Check sheet for the modelled part. Datum: model origin and axes. Units: mm. A direction names the side the tool comes from. Round coordinates to 2 decimals unless told otherwise and drop trailing zeros. Order: outer loops, then holes, each group sorted by start corner. A loop starts at its lowest first (then second) coordinate and runs counter-clockwise, first axis right, second up. Notation, with made-up numbers: (32.25, -36.5) -> (64.25, -36.5) arc R24 ccw to (64.25, -7.5) -> close; hole circle Ø5 at (60.25, -34). An arc over 180 degrees is marked (long way). Answer as CSV lines item,"result". Start each with the question number.
from build123d import *

# Parameters (mm, degrees)
SKICA1_W                 = 120
SKICA1_H                 = 75
P_IDAT_VYSUNUT_M9_DEPTH  = 7
SKICA9_W                 = 60
SKICA9_H                 = 75
P_IDAT_VYSUNUT_M10_DEPTH = 7
SKICA10_W                = 60
SKICA10_H                = 75
P_IDAT_VYSUNUT_M11_DEPTH = 7
SKICA11_W                = 120
SKICA11_H                = 60
P_IDAT_VYSUNUT_M12_DEPTH = 7
SKICA12_W                = 120
SKICA12_H                = 60
P_IDAT_VYSUNUT_M13_DEPTH = 7
SKICA13_R                = 1.75
SKICA13_W                = 7.3
SKICA13_H                = 8.5
ODEBRAT_VYSUNUT_M1_DEPTH = 7


with BuildPart() as part:
    # Skica1 → Přidat vysunutím9 (new body)
    with BuildSketch(Plane.XY):
        Rectangle(SKICA1_W, SKICA1_H)
    extrude(amount=P_IDAT_VYSUNUT_M9_DEPTH)

    # Skica9 → Přidat vysunutím10 (add)
    with BuildSketch(Plane.ZY.offset(60)):
        with Locations((30, 0)):
            Rectangle(SKICA9_W, SKICA9_H)
    extrude(amount=-P_IDAT_VYSUNUT_M10_DEPTH)

    # Skica10 → Přidat vysunutím11 (add)
    with BuildSketch(Plane(origin=(60, 0, 0), x_dir=(0, 0, -1), z_dir=(1, 0, 0))):
        with Locations((-30, 0)):
            Rectangle(SKICA10_W, SKICA10_H)
    extrude(amount=-P_IDAT_VYSUNUT_M11_DEPTH)

    # Skica11 → Přidat vysunutím12 (add)
    with BuildSketch(Plane(origin=(0, -37.5, 0), x_dir=(-1, 0, 0), z_dir=(0, -1, 0))):
        with Locations((0, -30)):
            Rectangle(SKICA11_W, SKICA11_H)
    extrude(amount=-P_IDAT_VYSUNUT_M12_DEPTH)

    # Skica12 → Přidat vysunutím13 (add)
    with BuildSketch(Plane(origin=(0, 37.5, 0), x_dir=(1, 0, 0), z_dir=(0, 1, 0))):
        with Locations((0, -30)):
            Rectangle(SKICA12_W, SKICA12_H)
    extrude(amount=-P_IDAT_VYSUNUT_M13_DEPTH)

    # Skica13 → Odebrat vysunutím1 (cut)
    with BuildSketch(Plane.ZY.offset(60)):
        with Locations(Location((41.3, 13.25, 0), (0, 0, 270))):
            Circle(SKICA13_R)
        with Locations((12.65, 13.25)):
            Rectangle(SKICA13_W, SKICA13_H)
    extrude(amount=-ODEBRAT_VYSUNUT_M1_DEPTH, mode=Mode.SUBTRACT)


solid = part.part
1) Depth check by flat-ended pin: pin 1 Ø18.5 at (x, y) = (-18.5, -3.5) entering from +Z. Enter the tip coordinate at first touch or a pass-through.
2) Section check D-D on x = -38. Record the cut outline in (y, z), then the cut area to 3 significant figures.
3) Section check C-C on y = 13.25. Record the cut outline in (x, z), then the cut area to 3 significant figures.
4) Section check A-A on y = -2.5. Record the cut outline in (x, z).
5) Mould release check, pull along Y, two halves, no side actions. Record for faces 4 (the face through (1, 37.5, 30)), 5 (the face through (1, -37.5, 30)), 6 (the face through (0, -31, 60)), 7 (the face through (1, -30.5, 33)): released by +Y, released by -Y, zero draft, split by the parting line, or undercut.
6) Access from +Z, -Z, +X, -X, +Y, -Y to the whole of each face (thin tool, end or side, straight path). Record for faces 1 (the face through (-60, -1, 30)), 2 (the face through (-57, 13, 9)), 3 (the face through (53, 0, 34)).
7) Material ranges on line 1 along Z through (x, y) = (-56, 13); line 2 along Y through (x, z) = (-33, 20); line 3 along X through (y, z) = (-29, 16), recorded low to high.
8) Section check B-B on z = 25. Record the cut outline in (x, y), then the cut area to 3 significant figures.
Solutions:
1,pin 1,"stops at z = 7"
2,outline,"(-37.5, 0) -> (37.5, 0) -> (37.5, 60) -> (30.5, 60) -> (30.5, 7) -> (-30.5, 7) -> (-30.5, 60) -> (-37.5, 60) -> close"
2,area,"1,270 mm^2"
3,outline,"(-60, 0) -> (60, 0) -> (60, 60) -> (53, 60) -> (53, 7) -> (-53, 7) -> (-53, 9) -> (-60, 9) -> close; (-60, 16.3) -> (-53, 16.3) -> (-53, 39.55) -> (-60, 39.55) -> close; (-60, 43.05) -> (-53, 43.05) -> (-53, 60) -> (-60, 60) -> close"
3,area,"1,510 mm^2"
4,outline,"(-60, 0) -> (60, 0) -> (60, 60) -> (53, 60) -> (53, 7) -> (-53, 7) -> (-53, 60) -> (-60, 60) -> close"
5,face 4,"released by +Y"
5,face 5,"released by -Y"
5,face 6,"zero draft"
5,face 7,"undercut"
6,face 1,"+Z, -Z, -X, +Y, -Y"
6,face 2,"-X"
6,face 3,"+Z"
7,line 1,"z = 0 to 9, 16.3 to 39.57, 43.03 to 60"
7,line 2,"y = -37.5 to -30.5, 30.5 to 37.5"
7,line 3,"x = -60 to -53, 53 to 60"
8,outline,"(-60, -37.5) -> (60, -37.5) -> (60, 37.5) -> (-60, 37.5) -> close; hole (-53, -30.5) -> (53, -30.5) -> (53, 30.5) -> (-53, 30.5) -> close"
8,area,"2,530 mm^2"
